Input: part model. Units: mm. Frame: model coordinates. Face numbers are marked on the shaded views. Give positions to 0.01 mm unless a question says otherwise; leave off trailing zeros. Order: outer loops, then holes, each group sorted by start corner. A loop starts at its lowest first (then second) coordinate and runs counter-clockwise, first axis right, second up.
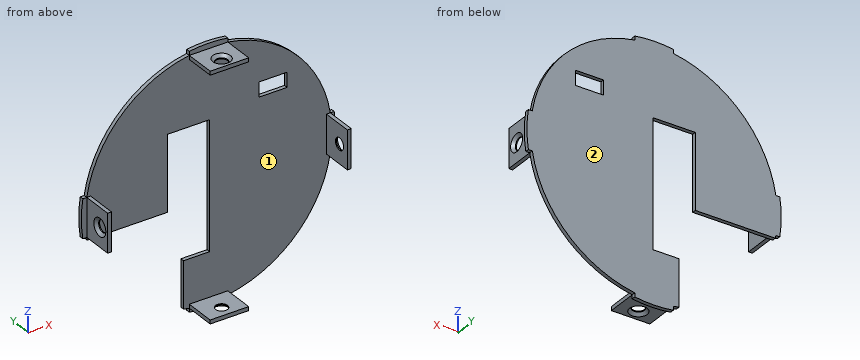
Autodesk Inventor part; units mm, degrees
ref_plane "Work Plane1" through (0, 1, 0) normal (0, 1, 0) x (1, 0, 0)
ref_plane "YZ Plane" through (0, 0, 0) normal (1, 0, 0) x (0, 1, 0)
ref_plane "XZ Plane" through (0, 0, 0) normal (0, 1, 0) x (-1, 0, 0)
sketch "Sketch1" plane through (0, 0, 0) normal (0, 1, 0) x (-1, 0, 0)
  arc A0 (31.6389, 4.7938) -> (6.5, -31.3329) centre (0, 0) ccw
  line L0 (-5, 33) -> (5, 33)
  line L1 (5, 33) -> (5, 31.607)
  line L2 (5, -33) -> (-5, -33)
  line L3 (-5, -33) -> (-5, 5)
  line L4 (-5, 33) -> (5, -33) construction
  line L5 (5, 33) -> (-5, -33) construction
  line L6 (-33, 5) -> (-5, 5)
  line L7 (33, 5) -> (33, -5)
  line L8 (33, -5) -> (31.607, -5)
  line L9 (-33, -5) -> (-33, 5)
  line L10 (-33, 5) -> (33, -5) construction
  line L11 (33, 5) -> (-33, -5) construction
  arc A1 (4.7938, -31.6389) -> (6.5, -31.3329) centre (0, 0) ccw
  line L12 (6.5, -31.3329) -> (6.5, -19.2329)
  line L13 (6.5, -19.2329) -> (-0.3, -19.2329)
  line L14 (-0.3, -19.2329) -> (-0.3, -5.7329)
  line L15 (-0.3, 13.7671) -> (5, 13.7671)
  line L16 (10.7, 13.7671) -> (10.7, 5)
  line L17 (10.7, -5.7329) -> (31.4823, -5.7329)
  arc A2 (31.4823, -5.7329) -> (31.607, -5) centre (0, 0) ccw
  arc A3 (31.6389, -4.7938) -> (31.6389, 4.7938) centre (0, 0) ccw
  line L18 (5, -19.2329) -> (5, -33)
  line L19 (5, 13.7671) -> (5, 5)
  line L20 (10.7, 1.6212) -> (10.7, -5.7329)
  line L21 (-0.3, -5) -> (-0.3, 5)
  arc A4 (6.5, -31.3329) -> (10.7, -30.1581) centre (0, 0) ccw
  line L22 (5, -5) -> (0.7576, -5)
  line L23 (5, 5) -> (10.7, 5)
  line L24 (-5, 5) -> (-0.3, 5)
  line L25 (-5, -5) -> (-33, -5)
  line L26 (-5, 5) -> (-5, 33)
  line L27 (5, 5) -> (5, -5)
  line L28 (5, 31.607) -> (5, 13.7671)
  arc A5 (10.7, -30.1581) -> (31.4823, -5.7329) centre (0, 0) ccw
  arc A6 (6.5, -31.3329) -> (31.6389, -4.7938) centre (0, 0) ccw
  line L29 (-0.3, -5.7329) -> (-0.3, -5)
  line L30 (5, -5) -> (5, -5.7329)
  line L31 (10.7, 5) -> (31.607, 5)
  line L32 (10.7, -5) -> (5, -5)
  line L33 (0.7576, 5) -> (5, 5)
  line L34 (-0.3, 5) -> (0.7576, 5)
  line L35 (5, 13.7671) -> (10.7, 13.7671)
  line L36 (-0.3, 5) -> (-0.3, 13.7671)
  line L37 (31.607, 5) -> (33, 5)
  line L38 (10.7, 5) -> (10.7, 1.6212)
  line L39 (31.607, -5) -> (10.7, -5)
  line L40 (0.7576, -5) -> (-5, -5)
  line L41 (5, -5.7329) -> (5, -19.2329)
  dimension "d0" = 64
  dimension "d1" = 10
  dimension "d2" = 66
  dimension "d3" = 66
  dimension "d4" = 10
  dimension "d11" = 12.1
  dimension "d12" = 6.8
  dimension "d13" = 33
  dimension "d14" = 0.3
  dimension "d15" = 11
  dimension "d16" = 19.5
ref_plane "Work Plane1" through (0, 1, 0) normal (0, 1, 0) x (1, 0, 0)
sketch "Sketch2" plane through (0, 1, 0) normal (0, 1, 0) x (1, 0, 0)
  circle A0 centre (0, 0) radius 33
  dimension "d7" = 66
extrude "Extrusion2" [suppressed]
extrude "Extrusion3" add sketch "Sketch1" along normal blind 1 contours A3 A6 L39 L20 L38 L31 A0 | A0 L37 L7 L8 A6 A3 | L31 L16 L35 L28 A0 | L28 L15 L36 L24 L26 A0 | A0 L26 L0 L1 | A2 L17 L20 L39 | L26 L6 A0 | L6 L3 L25 A0 | A0 L25 L9 L6 | L24 L21 L40 L3 | L25 L3 A0 | L40 L29 L14 L13 L18 A0 L3 | A0 L18 L13 L12 | A0 L18 L2 L3
sketch "Sketch3" plane through (0, 0, 0) normal (0, -1, 0) x (1, 0, 0)
  line L0 (-5, -33) -> (-5, -31.607)
  line L1 (-5, -31.607) -> (5, -31.607)
  line L2 (5, -31.607) -> (5, -30.607)
  line L3 (5, -30.607) -> (-5, -30.607)
  line L4 (-5, -30.607) -> (-5, -31.607)
  line L5 (-33, 5) -> (-31.607, 5)
  line L6 (-31.607, 5) -> (-30.607, 5)
  line L7 (-30.607, 5) -> (-30.607, -5)
  line L8 (-30.607, -5) -> (-31.607, -5)
  line L9 (-31.607, -5) -> (-31.607, 5)
  line L10 (-5, 31.607) -> (-5, 33)
  line L11 (-5, 31.607) -> (5, 31.607)
  line L12 (5, 31.607) -> (5, 30.607)
  line L13 (5, 30.607) -> (-5, 30.607)
  line L14 (-5, 30.607) -> (-5, 31.607)
  line L15 (31.607, 5) -> (30.607, 5)
  line L16 (30.607, 5) -> (30.607, -5)
  line L17 (30.607, -5) -> (31.607, -5)
  line L18 (31.607, -5) -> (31.607, 5)
  line L19 (31.607, 5) -> (33, 5)
  dimension "d21" = 10
  dimension "d22" = 1
  dimension "d23" = 1
  dimension "d24" = 10
  dimension "d25" = 10
  dimension "d26" = 1
  dimension "d27" = 1
  dimension "d28" = 10
extrude "Extrusion4" add sketch "Sketch3" along normal blind 8
sketch "Sketch4" plane through (31.607, 0, 5) normal (1, 0, 0) x (0, 0, -1)
  circle A0 centre (5, -5) radius 2.295
  line L0 (0, 0) -> (10, 0)
  point P0 (5, 0)
  point P1 (5, 0)
  dimension "d31" = 4.59
  dimension "d32" = 5
hole "Hole1" at (31.607, -5, 0) direction (-1, 0, 0) diameter 3.1 end through all countersink diameter 4.59 countersink angle 90
pattern_circular "Circular Pattern1" count 4 over 360 about axis through (0, 0, 0) along (0, 1, 0) of "Hole1"
sketch "Sketch5" plane through (0, 1, 0) normal (0, 1, 0) x (1, 0, 0)
  circle A0 centre (0, 0) radius 33
  dimension "d43" = 66
extrude "Extrusion5" cut sketch "Sketch5" against normal blind 100 keep common part
sketch "Sketch6" plane through (0, 1, 0) normal (0, 1, 0) x (1, 0, 0)
  arc A0 (5, -31.607) -> (31.607, -5) centre (0, 0) ccw
  line L0 (5, -31.607) -> (5, -18.907)
  line L1 (31.607, -5) -> (20.407, -5)
  line L2 (20.407, -5) -> (20.407, -18.907)
  line L3 (20.407, -18.907) -> (5, -18.907)
  line L4 (13.107, -18.907) -> (20.407, -18.907)
  line L5 (20.407, -18.907) -> (20.407, -15.107)
  line L6 (20.407, -15.107) -> (13.107, -15.107)
  line L7 (13.107, -15.107) -> (13.107, -18.907)
  dimension "d46" = 12.7
  dimension "d47" = 11.2
  dimension "d48" = 7.3
  dimension "d49" = 3.8
extrude "Extrusion6" cut sketch "Sketch6" against normal blind 10 contours L7 L6 L2 L3
properties part number "Hull_top"
1) First-contact query: P1, Ø3.5, axis at y = -5, z = 0, coming from the -X side; P2, Ø3, axis at x = -18.5, z = -6.5, coming from the -Y side; P3, Ø0.6, axis at x = 31.5, y = -3.5, coming from the -Z side. Flat tips, straight axial feed; report the tip coordinate or a pass-through.
2) Line query: probe 1 along Y at (x, z) = (30.85, 0); probe 2 along Z at (x, y) = (4, -7); probe 3 along Y at (x, z) = (10, -4.5). Output: solid intervals per line, ascending.
3) Cut plane B-B (y = -5). Count the separate pieces of the cut face and the enclosed holes in it, then the cut area to 3 significant figures.
4) Cut plane A-A (z = 0). Return the cut outline in (x, y) (3 decimals), then the cut area to 3 significant figures.
5) Pull-direction query (Z, two-part tool) for the marked faces 1 and 2; classes: pulls with the +Z half, pulls with the -Z half, needs draft (parallel to the pull), parting line crosses it, or undercut.
6) Cut plane C-C (x = -24.5). Return the cut outline in (y, z), then the cut area to 3 significant figures.
7) Cut plane D-D (z = 22.5). Return the cut outline in (x, y), then the cut area to 3 significant figures.
Geometry says:
1. P1: stops at x = -31.06
1. P2: stops at y = 0
1. P3: stops at z = -5
2. probe 1: y = -8 to -6.55, -3.45 to 1
2. probe 2: z = -31.61 to -30.61, 30.61 to 31.61
2. probe 3: y = 0 to 1
3. separate pieces: 8
3. enclosed holes: 0
3. area: 25.4 mm2
4. outline: (-33, 0) - (-31.607, 0) - (-31.607, -2.705) - (-30.862, -3.45) - (-30.607, -3.45) - (-30.607, 0) - (-10.7, 0) - (-10.7, 1) - (-33, 1) - close; (-31.607, -8) - (-30.607, -8) - (-30.607, -6.55) - (-30.862, -6.55) - (-31.607, -7.295) - close; (0.3, 0) - (30.607, 0) - (30.607, -3.45) - (30.862, -3.45) - (31.607, -2.705) - (31.607, 0) - (33, 0) - (33, 1) - (0.3, 1) - close; (30.607, -8) - (31.607, -8) - (31.607, -7.295) - (30.862, -6.55) - (30.607, -6.55) - close
4. area: 63.7 mm2
5. face 1: undercut
5. face 2: needs draft
6. outline: (0, -5.73) - (1, -5.73) - (1, 20.59) - (0, 20.59) - close
6. area: 26.3 mm2
7. outline: (-22.75, 0) - (22.75, 0) - (22.75, 1) - (-22.75, 1) - close
7. area: 45.5 mm2
